```python
from build123d import *

# Parameters (mm, degrees)
F0_W      = 111.125
F0_H      = 102.616
F1_DEPTH  = 1.99898
F2_W      = 55.88
F2_H      = 54.61
F3_DEPTH  = 1.10998
F4_W      = 77.216
F4_H      = 89.916
F5_DEPTH  = 0.889
F6_W      = 76.2
F6_H      = 88.9
F7_DEPTH  = 0.65024
F8_W      = 56.388
F8_H      = 56.388
F9_DEPTH  = 0.65024
F10_W     = 63.99276
F10_H     = 64.36106
F11_DEPTH = 0.59944
F12_W     = 104.648
F12_H     = 101.6
F13_DEPTH = 0.254


with BuildPart() as f1:
    # F0 (on Front) → F1 (new body)
    with BuildSketch(Plane.XZ):
        with Locations((-8.899393, -4.392473)):
            Rectangle(F0_W, F0_H)
    extrude(amount=F1_DEPTH)

    # F2 (on face) → F3 (cut)
    with BuildSketch(Plane.XZ.offset(1.99898)):
        with Locations((2.314707, -4.392473)):
            Rectangle(F2_W, F2_H)
    extrude(amount=-F3_DEPTH, mode=Mode.SUBTRACT)

    # F4 (on face) → F5 (cut)
    with BuildSketch(Plane(origin=(0, 0, 0), x_dir=(-1, 0, 0), z_dir=(0, 1, 0))):
        with Locations((-2.975107, -4.392473)):
            Rectangle(F4_W, F4_H)
    extrude(amount=-F5_DEPTH, mode=Mode.SUBTRACT)

    # F6 (on face) → F7 (join)
    with BuildSketch(Plane(origin=(0, -0.889, 0), x_dir=(-1, 0, 0), z_dir=(0, 1, 0))):
        with Locations((-3.483107, -3.884473)):
            Rectangle(F6_W, F6_H)
    extrude(amount=F7_DEPTH)

    # F8 (on face) → F9 (cut)
    with BuildSketch(Plane(origin=(0, -0.23876, 0), x_dir=(-1, 0, 0), z_dir=(0, 1, 0))):
        with Locations((-2.975107, -3.884473)):
            Rectangle(F8_W, F8_H)
    extrude(amount=-F9_DEPTH, mode=Mode.SUBTRACT)

    # F10 (on face) → F11 (join)
    with BuildSketch(Plane(origin=(0, -0.23876, 0), x_dir=(-1, 0, 0), z_dir=(0, 1, 0))):
        with Locations((-2.975107, -4.393743)):
            Rectangle(F10_W, F10_H)
    extrude(amount=F11_DEPTH)

    # F12 (on face) → F13 (join)
    with BuildSketch(Plane(origin=(0, 0, 0), x_dir=(-1, 0, 0), z_dir=(0, 1, 0))):
        with Locations((16.849593, -3.884473)):
            Rectangle(F12_W, F12_H)
    extrude(amount=F13_DEPTH)


solid = f1.part
```
Build history of the part. All positions in model axes, mm. A direction names the side the tool comes from. Give positions to 0.01 mm unless a question says otherwise; leave off trailing zeros. Loops run counter-clockwise (first coordinate to the right, second up) from the corner with the lowest first, then second, coordinate; pieces in that order, holes last.
1) Two-plate mould, pull along Z, no slides. Class faces 4 (the face through (15.6, -0.889, 23.4)), 5 (the face through (44, 0, -4)): released by +Z, released by -Z, zero draft, split by the parting line, or undercut.
Values follow:
face 4: undercut
face 5: zero draft
2) Band-saw the part on B-B on x = 24. List the corners of the cut face in (y, z), then the cut area to 3 significant figures.
Values follow:
outline: (-2, -55.7) - (0, -55.7) - (0, -54.68) - (0.25, -54.68) - (0.25, -36.57) - (0.36, -36.57) - (0.36, 27.79) - (0.25, 27.79) - (0.25, 46.92) - (-2, 46.92) - (-2, 22.91) - (-0.89, 22.91) - (-0.89, 24.31) - (-0.24, 24.31) - (-0.24, -32.08) - (-0.89, -32.08) - (-0.89, -31.7) - (-2, -31.7) - close; hole (-0.89, -49.35) - (0, -49.35) - (0, -36.57) - (-0.24, -36.57) - (-0.24, -48.33) - (-0.89, -48.33) - close; hole (-0.24, 27.79) - (0, 27.79) - (0, 40.57) - (-0.24, 40.57) - close
area: 134 mm2
3) 3-axis set-ups, long thin cutter, end or side, ignore diameter. For faces 1 (the face through (-67, 0, -3)), 2 (the face through (-34, -1.999, -4)), 3 (the face through (38, -0.239, -3)): which of +Z, -Z, +X, -X, +Y, -Y reach the whole face in a straight line?
Values follow:
face 1: +Z, -Z, -X, -Y
face 2: +Z, -Z, +X, -X, -Y
face 3: none
4) Probe line 1 along Z through (x, y) = (12, -0.4); line 2 along X through (y, z) = (-0.45, -8.5); line 3 along X through (y, z) = (-0.05, -34). List the from-to ranges inside material, lowest first.
Values follow:
line 1: z = -55.7 to -49.35, -48.33 to -32.08, 24.31 to 46.92
line 2: x = -64.46 to -35.63, -34.62 to -25.22, 31.17 to 46.66
line 3: x = -64.46 to -35.63, -29.02 to 34.97, 41.58 to 46.66
5) Band-saw the part on D-D on x = -33. List the corners of the cut face in (y, z), then the cut area to 3 significant figures.
Values follow:
outline: (-2, -55.7) - (0, -55.7) - (0, -54.68) - (0.25, -54.68) - (0.25, 46.92) - (-2, 46.92) - close; hole (-0.89, -49.35) - (0, -49.35) - (0, 40.57) - (-0.24, 40.57) - (-0.24, -48.33) - (-0.89, -48.33) - close
area: 209 mm2
6) Band-saw the part on C-C on y = -1.4. List the corners of the cut face in (x, z), then the cut area to 3 significant figures.
Values follow:
outline: (-64.46, -55.7) - (46.66, -55.7) - (46.66, 46.92) - (-64.46, 46.92) - close; hole (-25.63, -31.7) - (30.25, -31.7) - (30.25, 22.91) - (-25.63, 22.91) - close
area: 8,350 mm2
7) Drop flat-ended pins along their axis: P1, Ø0.6, axis at y = -1, z = -5, coming from the -X side; P2, Ø6, axis at x = -50.5, z = -45, coming from the +Y side. Give the stop position or say it passes through.
Values follow:
P1: stops at x = -64.46
P2: stops at y = 0.25
